```python
from build123d import *

# Parameters (mm, degrees)
SKETCH_1_W                   = 114
SKETCH_1_H                   = 200
EXTRUDE_1_DEPTH              = 15
HOLE_WIZARD_M4_1_D           = 4.5
HOLE_WIZARD_M4_1_CBORE_D     = 8
HOLE_WIZARD_M4_1_CBORE_DEPTH = 4.4
PATTERN_LINEAR_1_COUNT       = 2
PATTERN_LINEAR_1_PITCH       = 118
PATTERN_LINEAR_1_COUNT_DIR2  = 2
PATTERN_LINEAR_1_PITCH_DIR2  = 80
PATTERN_LINEAR_3_COUNT       = 2
PATTERN_LINEAR_3_PITCH       = 100
PATTERN_LINEAR_3_COUNT_DIR2  = 2
PATTERN_LINEAR_3_PITCH_DIR2  = 62


with BuildPart() as part:
    # 草图1 → 凸台-拉伸1 (new body)
    with BuildSketch(Plane(origin=(0, 0, 0), x_dir=(1, 0, 0), z_dir=(0, 1, 0))):
        Rectangle(SKETCH_1_W, SKETCH_1_H)
    extrude(amount=EXTRUDE_1_DEPTH)

    # Hole Wizard M4 _1 (through all)
    with Locations(Plane(origin=(0, 15, 0), x_dir=(1, 0, 0), z_dir=(0, 1, 0))):
        with Locations((-40, -90)):
            hole_wizard_m4_1 = CounterBoreHole(HOLE_WIZARD_M4_1_D / 2, HOLE_WIZARD_M4_1_CBORE_D / 2, HOLE_WIZARD_M4_1_CBORE_DEPTH)

    # 阵列(线性)1: Hole Wizard M4 _1 2 × 2
    with Locations(*[(j * PATTERN_LINEAR_1_PITCH_DIR2, 0, -i * PATTERN_LINEAR_1_PITCH) for i in range(PATTERN_LINEAR_1_COUNT) for j in range(PATTERN_LINEAR_1_COUNT_DIR2) if (i, j) != (0, 0)]):
        add(hole_wizard_m4_1, mode=Mode.SUBTRACT)

    # 草图6 → Hole Wizard M4 _1 2 (revolve, cut)
    with BuildSketch(Plane(origin=(-31, 15, 50), x_dir=(0, 0, 1), z_dir=(1, 0, 0))):
        Polygon((0, 0), (0, 11.091420021), (1.65, 10.1), (1.65, 0), align=None)
    hole_wizard_m4_1_2 = revolve(axis=Axis((-31, 21.35, 50), (0, -1, 0)), mode=Mode.SUBTRACT)

    # 阵列(线性)3: Hole Wizard M4 _1 2 2 × 2
    with Locations(*[(j * PATTERN_LINEAR_3_PITCH_DIR2, 0, -i * PATTERN_LINEAR_3_PITCH) for i in range(PATTERN_LINEAR_3_COUNT) for j in range(PATTERN_LINEAR_3_COUNT_DIR2) if (i, j) != (0, 0)]):
        add(hole_wizard_m4_1_2, mode=Mode.SUBTRACT)


solid = part.part
```
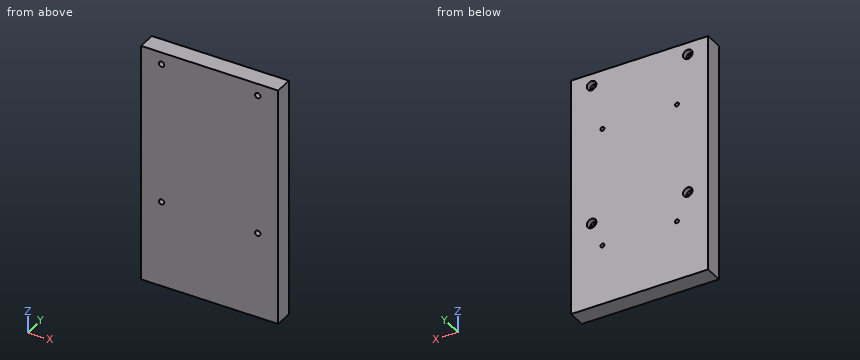
Source: CAD feature listing. Evaluate the final solid. Frame: model axes, mm. Give positions to 0.01 mm unless a question says otherwise; leave off trailing zeros. Write each loop counter-clockwise with the first axis right and the second up, starting at its lowest first coordinate (ties: lowest second). Pieces come first, ordered by that corner, then holes.
1. Material intervals for line 1 along X through (y, z) = (7.75, -50); line 2 along X through (y, z) = (13.1, 90); line 3 along Z through (x, y) = (-42, 13.5), sorted ascending.
2. Section query B-B (z = 90). Return the cut outline in (x, y).
3. Section query A-A (x = -40). Return the cut outline in (y, z).
4. First-contact query: pin 1 (3 mm diameter, centred on x = -31, z = 50, fed in from +Y); pin 2 (2.5 mm diameter, centred on x = 38.5, z = 90, fed in from +Y); pin 3 (2 mm diameter, centred on x = 31, z = 50, fed in from +Y). Flat tips, straight axial feed; report the tip coordinate or a pass-through.
Output values:
1. line 1: x = -57 to -32.65, -29.35 to 29.35, 32.65 to 57
1. line 2: x = -57 to -44, -36 to 36, 44 to 57
1. line 3: z = -100 to -31.46, -24.54 to 86.54, 93.46 to 100
2. outline: (-57, 0) - (-42.25, 0) - (-42.25, 10.6) - (-44, 10.6) - (-44, 15) - (-57, 15) - close; (-37.75, 0) - (37.75, 0) - (37.75, 10.6) - (36, 10.6) - (36, 15) - (-36, 15) - (-36, 10.6) - (-37.75, 10.6) - close; (42.25, 0) - (57, 0) - (57, 15) - (44, 15) - (44, 10.6) - (42.25, 10.6) - close
3. outline: (0, -100) - (15, -100) - (15, -32) - (10.6, -32) - (10.6, -30.25) - (0, -30.25) - close; (0, -25.75) - (10.6, -25.75) - (10.6, -24) - (15, -24) - (15, 86) - (10.6, 86) - (10.6, 87.75) - (0, 87.75) - close; (0, 92.25) - (10.6, 92.25) - (10.6, 94) - (15, 94) - (15, 100) - (0, 100) - close
4. pin 1: stops at y = 4.81
4. pin 2: stops at y = 10.6
4. pin 3: stops at y = 4.51
